Work out the finished part from the listing and answer in its coordinate system (mm). A direction names the side the tool comes from. Coordinates: 2 decimals unless noted, no trailing zeros. Loops run counter-clockwise (first coordinate to the right, second up) from the corner with the lowest first, then second, coordinate; pieces in that order, holes last. Notation, with made-up numbers: (-2, -28.75) - (53, -28.75) arc R17 ccw to (53, -3.75) - close; hole circle Ø8 at (-32.5, 26.5). An arc over 180 degrees is marked (long way). Write each question's results on one line, items separated by ' | '. Start each with the question number.
1. A cutting plane is placed at A-A on y = 14. Determine the outline of the cut face in (x, z), then the cut area to 3 significant figures.
2. A cutting plane is placed at B-B on x = 0. Determine the outline of the cut face in (y, z), then the cut area to 3 significant figures.
3. Which of the six approach directions +Z, -Z, +X, -X, +Y, -Y give full straight-line access (tool end or side, diameter ignored) to faces 1 (the flat face through (1, 100, -21)), 2 (the flat face through (-5.021, 3, 60)), 3 (the flat face through (-21.15, 11, 0))?
4. Find the intervals of material crossed by line 1 along Z through (x, y) = (0, 56); line 2 along Y through (x, z) = (14, 9); line 3 along X through (y, z) = (10.5, -11), in increasing order. Write a range as [from, to].
5. Determine the mould class of faces 4 (the cylindrical face through (-95.38, 49.3, -30.04)), 5 (the cylindrical face through (-0.54, 61.47, -2.44)), 6 (the flat face through (0, 6, 61)) for opening direction Z: released by +Z, released by -Z, zero draft, split by the parting line, or undercut.
6. A cutting plane is placed at C-C on z = 0. Determine the outline of the cut face in (x, y).
7. A cutting plane is placed at D-D on y = 33. Determine the outline of the cut face in (x, z), then the cut area to 3 significant figures.
8. Each of these flat-tipped pins is pushed along its axis until it touches: P1, Ø1, axis at x = -17.5, z = -71.5, coming from the -Y side; P2, Ø10, axis at y = 72, z = 67.5, coming from the +X side; P3, Ø1.5, axis at y = 34, z = -3.5, coming from the -X side; P4, Ø6, axis at x = 1.5, z = 61.5, coming from the -Y side. Where does it stop, or does it pass through?
Autodesk Inventor part; units mm, degrees
ref_plane "YZ Plane" through (0, 0, 0) normal (1, 0, 0) x (0, 1, 0)
ref_plane "XZ Plane" through (0, 0, 0) normal (0, 1, 0) x (-1, 0, 0)
ref_plane "XY Plane" through (0, 0, 0) normal (0, 0, 1) x (1, 0, 0)
sketch "Sketch1" plane through (0, 0, 0) normal (0, 1, 0) x (-1, 0, 0)
  circle A0 centre (0, 0) radius 100
  dimension "d0" = 200
extrude "Extrusion1" add sketch "Sketch1" along normal blind 100
sketch "Sketch2" plane through (0, 100, 0) normal (0, 1, 0) x (1, 0, 0)
  circle A0 centre (0, 0) radius 2.5
  dimension "d3" = 5
extrude "Extrusion2" cut sketch "Sketch2" along normal blind 22
sketch "Sketch6" plane through (0, 0, 0) normal (0, -1, 0) x (1, 0, 0)
  line L0 (15.5, 15.5) -> (-15.5, 15.5)
  line L1 (-15.5, 15.5) -> (-15.5, -15.5)
  line L2 (-15.5, -15.5) -> (15.5, -15.5)
  line L3 (15.5, -15.5) -> (15.5, 15.5)
  line L4 (15.5, 15.5) -> (-15.5, -15.5) construction
  line L5 (-15.5, 15.5) -> (15.5, -15.5) construction
  line L6 (21.15, 21.15) -> (-21.15, 21.15)
  line L7 (-21.15, 21.15) -> (-21.15, -21.15)
  line L8 (-21.15, -21.15) -> (21.15, -21.15)
  line L9 (21.15, -21.15) -> (21.15, 21.15)
  line L10 (21.15, 21.15) -> (-21.15, -21.15) construction
  line L11 (-21.15, 21.15) -> (21.15, -21.15) construction
  circle A0 centre (-15.5, -15.5) radius 1.4
  circle A1 centre (-15.5, 15.5) radius 1.4
  circle A2 centre (15.5, 15.5) radius 1.4
  circle A3 centre (15.5, -15.5) radius 1.4
  point P0 (0, 0)
  dimension "d18" = 31
  dimension "d19" = 31
  dimension "d21" = 42.3
  dimension "d22" = 42.3
  dimension "d23" = 2.8
  dimension "d24" = 2.8
  dimension "d25" = 2.8
  dimension "d26" = 2.8
extrude "Extrusion5" cut sketch "Sketch6" against normal blind 22 contours L0 A2 L3 A3 L2 A0 L1 A1 | L9 L8 L7 L6
sketch "Sketch7" plane through (0, 22, 0) normal (0, -1, 0) x (1, 0, 0)
  circle A0 centre (0, 0) radius 2.5
  circle A1 centre (0, 0) radius 2.5
  dimension "d29" = 5
extrude "Extrusion6" cut sketch "Sketch7" against normal blind 80
sketch "Sketch8" plane through (0, 22, 0) normal (0, -1, 0) x (1, 0, 0)
  circle A0 centre (0, 0) radius 11
  dimension "d32" = 22
extrude "Extrusion7" cut sketch "Sketch8" against normal blind 2
sketch "Sketch9" plane through (0, 0, 0) normal (0, -1, 0) x (1, 0, 0)
  line L0 (-21.15, 21.15) -> (21.15, 21.15)
  circle A0 centre (0, 0) radius 100
  line L1 (5.3123, 21.15) -> (-5.021, 21.15)
  line L2 (-5.021, 99.8739) -> (5.3123, 99.8739)
  line L3 (-5.021, 21.15) -> (-0.021, 21.15)
  line L4 (-0.021, 99.8739) -> (-5.021, 99.8739)
  line L5 (5.3123, 21.15) -> (-5.021, 21.15)
  line L6 (-5.021, 21.15) -> (-5.021, 99.8739)
  line L7 (-5.021, 99.8739) -> (5.3123, 99.8739)
  line L8 (5.3123, 99.8739) -> (5.3123, 21.15)
  arc A1 (5.3123, 99.8739) -> (-5.021, 99.8739) centre (0.1457, 63.1234) ccw
  point P0 (5.021, 99.8739)
  point P1 (5.3123, 99.8588)
  dimension "d40" = 78.7239
extrude "Extrusion8" cut sketch "Sketch9" against normal blind 6 contours L6 L2 A0 L8 L0 | A1 L2 A0 | A0 L2
equation "\"d24\" = d23"
equation "\"d25\" = d23"
equation "\"d26\" = d23"
properties part number "Base"
Values:
1) outline: circle Ø200 at (0, 0); circle Ø2.8 at (-15.5, -15.5); circle Ø2.8 at (-15.5, 15.5); circle Ø2.8 at (15.5, -15.5); circle Ø2.8 at (15.5, 15.5); hole (-21.15, -21.15) - (21.15, -21.15) - (21.15, 21.15) - (-21.15, 21.15) - close | area: 29,700 mm^2
2) outline: (0, -100) - (100, -100) - (100, -2.5) - (24, -2.5) - (24, -11) - (22, -11) - (22, -21.15) - (0, -21.15) - close; (6, 21.15) - (22, 21.15) - (22, 11) - (24, 11) - (24, 2.5) - (100, 2.5) - (100, 100) - (6, 100) - close | area: 18,200 mm^2
3) face 1: +Z, -Z, +X, -X, +Y | face 2: +Z, -Y | face 3: -Y
4) line 1: [-100, -2.5], [2.5, 100] | line 2: [22, 100] | line 3: [-99.39, -21.15], [21.15, 99.39]
5) face 4: split by the parting line | face 5: undercut | face 6: zero draft
6) outline: (-100, 0) - (-21.15, 0) - (-21.15, 22) - (-11, 22) - (-11, 24) - (-2.5, 24) - (-2.5, 100) - (-100, 100) - close; (2.5, 24) - (11, 24) - (11, 22) - (21.15, 22) - (21.15, 0) - (100, 0) - (100, 100) - (2.5, 100) - close
7) outline: circle Ø200 at (0, 0); hole circle Ø5 at (0, 0) | area: 31,400 mm^2
8) P1: y = 0 | P2: x = 78.06 | P3: x = -99.96 | P4: y = 6
